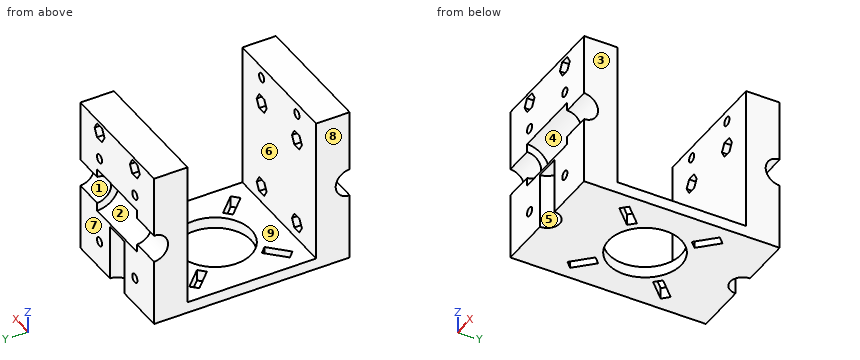
```python
from build123d import *

# Parameters (mm, degrees)
CYLINDER011_R           = 1.6
CYLINDER011_DEPTH       = 70
CYLINDER011_ROLL_ANGLE  = 90
CYLINDER010_R           = 1.6
CYLINDER010_DEPTH       = 70
CYLINDER010_ROLL_ANGLE  = 90
PRISM007_DEPTH          = 5
PRISM007_ROLL_ANGLE     = 90
PRISM006_DEPTH          = 5
PRISM006_ROLL_ANGLE     = 90
PRISM005_DEPTH          = 5
PRISM005_ROLL_ANGLE     = 90
PRISM004_DEPTH          = 5
PRISM004_ROLL_ANGLE     = 90
PRISM003_DEPTH          = 56
PRISM003_ROLL_ANGLE     = 90
PRISM002_DEPTH          = 56
PRISM002_ROLL_ANGLE     = 90
PRISM001_DEPTH          = 56
PRISM001_ROLL_ANGLE     = 90
PRISM_DEPTH             = 56
PRISM_ROLL_ANGLE        = 90
CYLINDER009_R           = 1.6
CYLINDER009_DEPTH       = 72
CYLINDER009_ROLL_ANGLE  = 90
CYLINDER008_R           = 1.6
CYLINDER008_DEPTH       = 72
CYLINDER008_ROLL_ANGLE  = 90
CYLINDER007_R           = 1.6
CYLINDER007_DEPTH       = 72
CYLINDER007_ROLL_ANGLE  = 90
CYLINDER006_R           = 1.6
CYLINDER006_DEPTH       = 72
CYLINDER006_ROLL_ANGLE  = 90
CYLINDER005_R           = 8
CYLINDER005_DEPTH       = 25
CYLINDER005_PITCH_ANGLE = 90
CYLINDER004_R           = 8
CYLINDER004_DEPTH       = 25
CYLINDER004_PITCH_ANGLE = 90
CYLINDER003_R           = 5
CYLINDER003_DEPTH       = 48
CYLINDER003_PITCH_ANGLE = 90
CYLINDER002_R           = 5
CYLINDER002_DEPTH       = 48
CYLINDER002_PITCH_ANGLE = 90
CYLINDER001_R           = 4.5
CYLINDER001_DEPTH       = 20
CYLINDER_R              = 4.5
CYLINDER_DEPTH          = 20
BOX001_W                = 46
BOX001_H                = 12
BOX001_DEPTH            = 56
BOX_W                   = 46
BOX_H                   = 12
BOX_DEPTH               = 56
SKETCH_W                = 46
SKETCH_H                = 70
SKETCH_R                = 13
PAD_DEPTH               = 4


with BuildPart() as cilindro011:
    # Cylinder011 → Cylinder011 (new body)
    with BuildSketch(Plane.XY):
        Circle(CYLINDER011_R)
    extrude(amount=CYLINDER011_DEPTH)


with BuildPart() as cilindro011_1:
    # Cylinder011 roll: moved
    add(cilindro011.part.rotate(Axis((0, 0, 0), (1, 0, 0)), CYLINDER011_ROLL_ANGLE))


with BuildPart() as cilindro011_2:
    # Cylinder011 placement: moved
    add(cilindro011_1.part.moved(Location((34, 70, 52))))


with BuildPart() as cilindro010:
    # Cylinder010 → Cylinder010 (new body)
    with BuildSketch(Plane.XY):
        Circle(CYLINDER010_R)
    extrude(amount=CYLINDER010_DEPTH)


with BuildPart() as cilindro010_1:
    # Cylinder010 roll: moved
    add(cilindro010.part.rotate(Axis((0, 0, 0), (1, 0, 0)), CYLINDER010_ROLL_ANGLE))


with BuildPart() as cilindro010_2:
    # Cylinder010 placement: moved
    add(cilindro010_1.part.moved(Location((12, 70, 52))))


with BuildPart() as prisma007:
    # Prism007 → Prism007 (new body)
    with BuildSketch(Plane.XY):
        Polygon((3.1, 0), (1.55, 2.684679), (-1.55, 2.684679), (-3.1, 0), (-1.55, -2.684679), (1.55, -2.684679), align=None)
    extrude(amount=PRISM007_DEPTH)


with BuildPart() as prisma007_1:
    # Prism007 roll: moved
    add(prisma007.part.rotate(Axis((0, 0, 0), (1, 0, 0)), PRISM007_ROLL_ANGLE))


with BuildPart() as prisma007_2:
    # Prism007 placement: moved
    add(prisma007_1.part.moved(Location((34, 70, 52))))


with BuildPart() as prisma006:
    # Prism006 → Prism006 (new body)
    with BuildSketch(Plane.XY):
        Polygon((3.1, 0), (1.55, 2.684679), (-1.55, 2.684679), (-3.1, 0), (-1.55, -2.684679), (1.55, -2.684679), align=None)
    extrude(amount=PRISM006_DEPTH)


with BuildPart() as prisma006_1:
    # Prism006 roll: moved
    add(prisma006.part.rotate(Axis((0, 0, 0), (1, 0, 0)), PRISM006_ROLL_ANGLE))


with BuildPart() as prisma006_2:
    # Prism006 placement: moved
    add(prisma006_1.part.moved(Location((12, 70, 52))))


with BuildPart() as prisma005:
    # Prism005 → Prism005 (new body)
    with BuildSketch(Plane.XY):
        Polygon((3.1, 0), (1.55, 2.684679), (-1.55, 2.684679), (-3.1, 0), (-1.55, -2.684679), (1.55, -2.684679), align=None)
    extrude(amount=PRISM005_DEPTH)


with BuildPart() as prisma005_1:
    # Prism005 roll: moved
    add(prisma005.part.rotate(Axis((0, 0, 0), (1, 0, 0)), PRISM005_ROLL_ANGLE))


with BuildPart() as prisma005_2:
    # Prism005 placement: moved
    add(prisma005_1.part.moved(Location((34, 5, 52))))


with BuildPart() as prisma004:
    # Prism004 → Prism004 (new body)
    with BuildSketch(Plane.XY):
        Polygon((3.1, 0), (1.55, 2.684679), (-1.55, 2.684679), (-3.1, 0), (-1.55, -2.684679), (1.55, -2.684679), align=None)
    extrude(amount=PRISM004_DEPTH)


with BuildPart() as prisma004_1:
    # Prism004 roll: moved
    add(prisma004.part.rotate(Axis((0, 0, 0), (1, 0, 0)), PRISM004_ROLL_ANGLE))


with BuildPart() as prisma004_2:
    # Prism004 placement: moved
    add(prisma004_1.part.moved(Location((12, 5, 52))))


with BuildPart() as prisma003:
    # Prism003 → Prism003 (new body)
    with BuildSketch(Plane.XY):
        Polygon((3.1, 0), (1.55, 2.684679), (-1.55, 2.684679), (-3.1, 0), (-1.55, -2.684679), (1.55, -2.684679), align=None)
    extrude(amount=PRISM003_DEPTH)


with BuildPart() as prisma003_1:
    # Prism003 roll: moved
    add(prisma003.part.rotate(Axis((0, 0, 0), (1, 0, 0)), PRISM003_ROLL_ANGLE))


with BuildPart() as prisma003_2:
    # Prism003 placement: moved
    add(prisma003_1.part.moved(Location((34, 63, 42))))


with BuildPart() as prisma002:
    # Prism002 → Prism002 (new body)
    with BuildSketch(Plane.XY):
        Polygon((3.1, 0), (1.55, 2.684679), (-1.55, 2.684679), (-3.1, 0), (-1.55, -2.684679), (1.55, -2.684679), align=None)
    extrude(amount=PRISM002_DEPTH)


with BuildPart() as prisma002_1:
    # Prism002 roll: moved
    add(prisma002.part.rotate(Axis((0, 0, 0), (1, 0, 0)), PRISM002_ROLL_ANGLE))


with BuildPart() as prisma002_2:
    # Prism002 placement: moved
    add(prisma002_1.part.moved(Location((12, 63, 42))))


with BuildPart() as prisma001:
    # Prism001 → Prism001 (new body)
    with BuildSketch(Plane.XY):
        Polygon((3.1, 0), (1.55, 2.684679), (-1.55, 2.684679), (-3.1, 0), (-1.55, -2.684679), (1.55, -2.684679), align=None)
    extrude(amount=PRISM001_DEPTH)


with BuildPart() as prisma001_1:
    # Prism001 roll: moved
    add(prisma001.part.rotate(Axis((0, 0, 0), (1, 0, 0)), PRISM001_ROLL_ANGLE))


with BuildPart() as prisma001_2:
    # Prism001 placement: moved
    add(prisma001_1.part.moved(Location((34, 63, 10))))


with BuildPart() as prisma:
    # Prism → Prism (new body)
    with BuildSketch(Plane.XY):
        Polygon((3.1, 0), (1.55, 2.684679), (-1.55, 2.684679), (-3.1, 0), (-1.55, -2.684679), (1.55, -2.684679), align=None)
    extrude(amount=PRISM_DEPTH)


with BuildPart() as prisma_1:
    # Prism roll: moved
    add(prisma.part.rotate(Axis((0, 0, 0), (1, 0, 0)), PRISM_ROLL_ANGLE))


with BuildPart() as prisma_2:
    # Prism placement: moved
    add(prisma_1.part.moved(Location((12, 63, 10))))


with BuildPart() as cilindro009:
    # Cylinder009 → Cylinder009 (new body)
    with BuildSketch(Plane.XY):
        Circle(CYLINDER009_R)
    extrude(amount=CYLINDER009_DEPTH)


with BuildPart() as cilindro009_1:
    # Cylinder009 roll: moved
    add(cilindro009.part.rotate(Axis((0, 0, 0), (1, 0, 0)), CYLINDER009_ROLL_ANGLE))


with BuildPart() as cilindro009_2:
    # Cylinder009 placement: moved
    add(cilindro009_1.part.moved(Location((34, 71, 42))))


with BuildPart() as cilindro008:
    # Cylinder008 → Cylinder008 (new body)
    with BuildSketch(Plane.XY):
        Circle(CYLINDER008_R)
    extrude(amount=CYLINDER008_DEPTH)


with BuildPart() as cilindro008_1:
    # Cylinder008 roll: moved
    add(cilindro008.part.rotate(Axis((0, 0, 0), (1, 0, 0)), CYLINDER008_ROLL_ANGLE))


with BuildPart() as cilindro008_2:
    # Cylinder008 placement: moved
    add(cilindro008_1.part.moved(Location((12, 71, 42))))


with BuildPart() as cilindro007:
    # Cylinder007 → Cylinder007 (new body)
    with BuildSketch(Plane.XY):
        Circle(CYLINDER007_R)
    extrude(amount=CYLINDER007_DEPTH)


with BuildPart() as cilindro007_1:
    # Cylinder007 roll: moved
    add(cilindro007.part.rotate(Axis((0, 0, 0), (1, 0, 0)), CYLINDER007_ROLL_ANGLE))


with BuildPart() as cilindro007_2:
    # Cylinder007 placement: moved
    add(cilindro007_1.part.moved(Location((34, 71, 10))))


with BuildPart() as cilindro006:
    # Cylinder006 → Cylinder006 (new body)
    with BuildSketch(Plane.XY):
        Circle(CYLINDER006_R)
    extrude(amount=CYLINDER006_DEPTH)


with BuildPart() as cilindro006_1:
    # Cylinder006 roll: moved
    add(cilindro006.part.rotate(Axis((0, 0, 0), (1, 0, 0)), CYLINDER006_ROLL_ANGLE))


with BuildPart() as cilindro006_2:
    # Cylinder006 placement: moved
    add(cilindro006_1.part.moved(Location((12, 71, 10))))


with BuildPart() as cilindro005:
    # Cylinder005 → Cylinder005 (new body)
    with BuildSketch(Plane.XY):
        Circle(CYLINDER005_R)
    extrude(amount=CYLINDER005_DEPTH)


with BuildPart() as cilindro005_1:
    # Cylinder005 pitch: moved
    add(cilindro005.part.rotate(Axis((0, 0, 0), (0, 1, 0)), CYLINDER005_PITCH_ANGLE))


with BuildPart() as cilindro005_2:
    # Cylinder005 placement: moved
    add(cilindro005_1.part.moved(Location((10.5, 70, 29))))


with BuildPart() as cilindro004:
    # Cylinder004 → Cylinder004 (new body)
    with BuildSketch(Plane.XY):
        Circle(CYLINDER004_R)
    extrude(amount=CYLINDER004_DEPTH)


with BuildPart() as cilindro004_1:
    # Cylinder004 pitch: moved
    add(cilindro004.part.rotate(Axis((0, 0, 0), (0, 1, 0)), CYLINDER004_PITCH_ANGLE))


with BuildPart() as cilindro004_2:
    # Cylinder004 placement: moved
    add(cilindro004_1.part.moved(Location((10.5, 0, 29))))


with BuildPart() as cilindro003:
    # Cylinder003 → Cylinder003 (new body)
    with BuildSketch(Plane.XY):
        Circle(CYLINDER003_R)
    extrude(amount=CYLINDER003_DEPTH)


with BuildPart() as cilindro003_1:
    # Cylinder003 pitch: moved
    add(cilindro003.part.rotate(Axis((0, 0, 0), (0, 1, 0)), CYLINDER003_PITCH_ANGLE))


with BuildPart() as cilindro003_2:
    # Cylinder003 placement: moved
    add(cilindro003_1.part.moved(Location((-1, 70, 29))))


with BuildPart() as cilindro002:
    # Cylinder002 → Cylinder002 (new body)
    with BuildSketch(Plane.XY):
        Circle(CYLINDER002_R)
    extrude(amount=CYLINDER002_DEPTH)


with BuildPart() as cilindro002_1:
    # Cylinder002 pitch: moved
    add(cilindro002.part.rotate(Axis((0, 0, 0), (0, 1, 0)), CYLINDER002_PITCH_ANGLE))


with BuildPart() as cilindro002_2:
    # Cylinder002 placement: moved
    add(cilindro002_1.part.moved(Location((-1, 0, 29))))


with BuildPart() as cilindro001:
    # Cylinder001 → Cylinder001 (new body)
    with BuildSketch(Plane(origin=(23, 70, 0), x_dir=(1, 0, 0), z_dir=(0, 0, 1))):
        Circle(CYLINDER001_R)
    extrude(amount=CYLINDER001_DEPTH)


with BuildPart() as cilindro:
    # Cylinder → Cylinder (new body)
    with BuildSketch(Plane(origin=(23, 0, 0), x_dir=(1, 0, 0), z_dir=(0, 0, 1))):
        Circle(CYLINDER_R)
    extrude(amount=CYLINDER_DEPTH)


with BuildPart() as cubo001:
    # Box001 → Box001 (new body)
    with BuildSketch(Plane(origin=(0, 58, 0), x_dir=(1, 0, 0), z_dir=(0, 0, 1))):
        with Locations((23, 6)):
            Rectangle(BOX001_W, BOX001_H)
    extrude(amount=BOX001_DEPTH)


with BuildPart() as cubo:
    # Box → Box (new body)
    with BuildSketch(Plane.XY):
        with Locations((23, 6)):
            Rectangle(BOX_W, BOX_H)
    extrude(amount=BOX_DEPTH)


with BuildPart() as cut019:
    # Sketch → Pad (new body)
    with BuildSketch(Plane.XY):
        with Locations((23, 35)):
            Rectangle(SKETCH_W, SKETCH_H)
        with Locations((23, 35)):
            Circle(SKETCH_R, mode=Mode.SUBTRACT)
        Polygon((39.19, 53.452742), (32.826039, 47.088781), (35.088781, 44.826039), (41.452742, 51.19), align=None, mode=Mode.SUBTRACT)
        Polygon((10.911219, 44.826039), (13.173961, 47.088781), (6.81, 53.452742), (4.547258, 51.19), align=None, mode=Mode.SUBTRACT)
        Polygon((4.547258, 18.81), (10.911219, 25.173961), (13.173961, 22.911219), (6.81, 16.547258), align=None, mode=Mode.SUBTRACT)
        Polygon((39.19, 16.547258), (32.826039, 22.911219), (35.088781, 25.173961), (41.452742, 18.81), align=None, mode=Mode.SUBTRACT)
    extrude(amount=PAD_DEPTH)

    # Fusion: union Cubo
    add(cubo.part)

    # Fusion001: union Cubo001
    add(cubo001.part)

    # Cut: cut Cilindro
    add(cilindro.part, mode=Mode.SUBTRACT)

    # Cut001: cut Cilindro001
    add(cilindro001.part, mode=Mode.SUBTRACT)

    # Cut002: cut Cilindro002
    add(cilindro002_2.part, mode=Mode.SUBTRACT)

    # Cut003: cut Cilindro003
    add(cilindro003_2.part, mode=Mode.SUBTRACT)

    # Cut004: cut Cilindro004
    add(cilindro004_2.part, mode=Mode.SUBTRACT)

    # Cut005: cut Cilindro005
    add(cilindro005_2.part, mode=Mode.SUBTRACT)

    # Cut006: cut Cilindro006
    add(cilindro006_2.part, mode=Mode.SUBTRACT)

    # Cut007: cut Cilindro007
    add(cilindro007_2.part, mode=Mode.SUBTRACT)

    # Cut008: cut Cilindro008
    add(cilindro008_2.part, mode=Mode.SUBTRACT)

    # Cut009: cut Cilindro009
    add(cilindro009_2.part, mode=Mode.SUBTRACT)

    # Cut010: cut Prisma
    add(prisma_2.part, mode=Mode.SUBTRACT)

    # Cut011: cut Prisma001
    add(prisma001_2.part, mode=Mode.SUBTRACT)

    # Cut012: cut Prisma002
    add(prisma002_2.part, mode=Mode.SUBTRACT)

    # Cut013: cut Prisma003
    add(prisma003_2.part, mode=Mode.SUBTRACT)

    # Cut014: cut Prisma004
    add(prisma004_2.part, mode=Mode.SUBTRACT)

    # Cut015: cut Prisma005
    add(prisma005_2.part, mode=Mode.SUBTRACT)

    # Cut016: cut Prisma006
    add(prisma006_2.part, mode=Mode.SUBTRACT)

    # Cut017: cut Prisma007
    add(prisma007_2.part, mode=Mode.SUBTRACT)

    # Cut018: cut Cilindro010
    add(cilindro010_2.part, mode=Mode.SUBTRACT)

    # Cut019: cut Cilindro011
    add(cilindro011_2.part, mode=Mode.SUBTRACT)


solid = cut019.part
```
Work out the finished part from the listing and answer in its coordinate system (mm). Face numbers are marked on the shaded views. A direction names the side the tool comes from. Round coordinates to 2 decimals unless told otherwise and drop trailing zeros. Loops run counter-clockwise (first coordinate to the right, second up) from the corner with the lowest first, then second, coordinate; pieces in that order, holes last. Notation, with made-up numbers: M 32,84 L 78,84 A22 ccw 78,115 Z; hole C 58.5,15 d2. An arc over 180 degrees is marked long. Use CSV: the item, a comma, the result in double quotes.
Q1. Section A-A, the plane y = 35 is taken. Determine the outline of the cut face in (x, z), then the cut area to 3 significant figures.
Determined:
outline,"M 0,0 L 10,0 L 10,4 L 0,4 Z; M 36,0 L 46,0 L 46,4 L 36,4 Z"
area,"80.0 mm2"
Q2. Section D-D, the plane y = 44 is taken. Determine the outline of the cut face in (x, z), then the cut area to 3 significant figures.
Determined:
outline,"M 0,0 L 13.62,0 L 13.62,4 L 0,4 Z; M 32.38,0 L 46,0 L 46,4 L 32.38,4 Z"
area,"109 mm2"
Q3. A tool of negligible diameter and unlimited length cuts with its end or side. For the marked faces 1, 2, 3, 4 and 5, from which of +Z, -Z, +X, -X, +Y, -Y can it reach the whole face along a straight path? Write none if from no direction.
Determined:
face 1,"+X, -X, +Y"
face 2,"+Y"
face 3,"+Z, -Z, +X, +Y, -Y"
face 4,"-Y"
face 5,"-Z, -Y"
Q4. Each of these flat-tipped pins is pushed along its axis until it touches: pin 1 (23.5 mm diameter, centred on x = 23, y = 35, fed in from -Z); pin 2 (1.5 mm diameter, centred on x = 26, z = 26, fed in from -Y); pin 3 (10 mm diameter, centred on x = 40.5, y = 19.5, fed in from +Z). Where does it stop, or does it pass through?
Determined:
pin 1,"through"
pin 2,"y = 7.07"
pin 3,"z = 4"
Q5. The mould has two halves that part along Y. Classify the marked faces 6, 7, 8 and 9: pulls with the +Y half, pulls with the -Y half, needs draft (parallel to the pull), parting line crosses it, or undercut.
Determined:
face 6,"undercut"
face 7,"pulls with the +Y half"
face 8,"needs draft"
face 9,"undercut"
Q6. Consider L1, parallel to X at y = 59, z = 52; L2, parallel to Z at x = 12, y = 61.25; L3, parallel to Y at x = 5.5, z = 40. Determine where each line is inside the solid, lowest interval first.
Determined:
L1,"0 to 10.4, 13.6 to 32.4, 35.6 to 46"
L2,"0 to 7.32, 12.68 to 39.32, 44.68 to 50.4, 53.6 to 56"
L3,"0 to 12, 58 to 70"
Q7. Section C-C, the plane z = 29 is taken. Determine the outline of the cut face in (x, y).
Determined:
outline,"M 0,5 L 10.5,5 L 10.5,8 L 35.5,8 L 35.5,5 L 46,5 L 46,12 L 0,12 Z; M 0,58 L 46,58 L 46,65 L 35.5,65 L 35.5,62 L 10.5,62 L 10.5,65 L 0,65 Z"
Q8. Section B-B, the plane x = 26.5 is taken. Determine the outline of the cut face in (y, z), then the cut area to 3 significant figures.
Determined:
outline,"M 0,20 L 2.83,20 L 2.83,0 L 22.48,0 L 22.48,4 L 12,4 L 12,56 L 0,56 L 0,37 A8 cw 0,21 Z; M 47.52,0 L 67.17,0 L 67.17,20 L 70,20 L 70,21 A8 cw 70,37 L 70,56 L 58,56 L 58,4 L 47.52,4 Z"
area,"1,110 mm2"
